```python
from build123d import *

# Parameters (mm, degrees)
CROQUIS1_W     = 15
CROQUIS1_H     = 65
EXTRUIR1_DEPTH = 6
CROQUIS2_W     = 15
CROQUIS2_H     = 6
EXTRUIR2_DEPTH = 50
CHAFL_N1_SIZE  = 2
CROQUIS3_R     = 4
EXTRUIR3_DEPTH = 50
CHAFL_N2_SIZE  = 3
REDONDEO1_R    = 6
CROQUIS4_R     = 4
EXTRUIR4_DEPTH = 30
REDONDEO2_R    = 0.5
EXTRUIR5_DEPTH = 15
CHAFL_N3_SIZE  = 9
EXTRUIR6_DEPTH = 15
CHAFL_N4_SIZE  = 3


with BuildPart() as part:
    # Croquis1 → Extruir1 (new body)
    with BuildSketch(Plane.XY):
        Rectangle(CROQUIS1_W, CROQUIS1_H)
    extrude(amount=EXTRUIR1_DEPTH)

    # Croquis2 → Extruir2 (add)
    with BuildSketch(Plane(origin=(0, 0, 0), x_dir=(-1, 0, 0), z_dir=(0, 0, -1))):
        with Locations((0, 29.5)):
            Rectangle(CROQUIS2_W, CROQUIS2_H)
    extrude(amount=EXTRUIR2_DEPTH)

    # Chaflán1
    chafl_n1_edges = [part.edges().sort_by_distance(p)[0] for p in [
        (0, 32.5, 6),
        (0, 26.5, 0),
    ]]
    chamfer(chafl_n1_edges, length=CHAFL_N1_SIZE)

    # Croquis3 → Extruir3 (add)
    with BuildSketch(Plane(origin=(0, 0, 0), x_dir=(-1, 0, 0), z_dir=(0, 0, -1))):
        with Locations(Location((0, -25.5, 0), (0, 0, 180))):
            Circle(CROQUIS3_R)
    extrude(amount=EXTRUIR3_DEPTH)

    # Chaflán2
    chafl_n2_edges = [part.edges().sort_by_distance(p)[0] for p in [
        (-4, -25.5, 0),
    ]]
    chamfer(chafl_n2_edges, length=CHAFL_N2_SIZE - 0.0001)  # a hair under: the kernel refuses the full size

    # Redondeo1
    redondeo1_edges = [part.edges().sort_by_distance(p)[0] for p in [
        (-7.5, -32.5, 3),
        (7.5, -32.5, 3),
    ]]
    fillet(redondeo1_edges, radius=REDONDEO1_R)

    # Croquis4 → Extruir4 (add)
    with BuildSketch(Plane(origin=(0, 32.5, 0), x_dir=(1, 0, 0), z_dir=(0, 1, 0))):
        with Locations(Location((0, 23, 0), (0, 0, 90))):
            Circle(CROQUIS4_R)
    extrude(amount=EXTRUIR4_DEPTH)

    # Redondeo2
    redondeo2_edges = [part.edges().sort_by_distance(p)[0] for p in [
        (0, 32.5, -19),
    ]]
    fillet(redondeo2_edges, radius=REDONDEO2_R)

    # Croquis6 → Extruir5 (add)
    with BuildSketch(Plane.XY.offset(6)):
        with BuildLine():
            Line((7.5, 0), (-7.5, 0))
            Line((-7.5, 0), (-7.5, -26.5))
            ThreePointArc((-7.5, -26.5), (-5.742640687, -30.742640687), (-1.5, -32.5))
            Line((-1.5, -32.5), (1.5, -32.5))
            ThreePointArc((1.5, -32.5), (5.742640687, -30.742640687), (7.5, -26.5))
            Line((7.5, -26.5), (7.5, 0))
        make_face()
    extrude(amount=-EXTRUIR5_DEPTH)

    # Chaflán3
    chafl_n3_edges = [part.edges().sort_by_distance(p)[0] for p in [
        (0, 0, 0),
    ]]
    chamfer(chafl_n3_edges, length=CHAFL_N3_SIZE - 0.0001)  # a hair under: the kernel refuses the full size

    # Croquis7 → Extruir6 (cut)
    with BuildSketch(Plane(origin=(7.5, 0, 0), x_dir=(0, 0, -1), z_dir=(1, 0, 0))):
        Polygon((-6, 6.514718626), (3, -2.485281374), (3, -32.5), (-11.901527466, -39.580751492), align=None)
    extrude(amount=-EXTRUIR6_DEPTH, mode=Mode.SUBTRACT)

    # Chaflán4
    chafl_n4_edges = [part.edges().sort_by_distance(p)[0] for p in [
        (-4, -25.5, -9),
    ]]
    chamfer(chafl_n4_edges, length=CHAFL_N4_SIZE - 0.0001)  # a hair under: the kernel refuses the full size


solid = part.part
```
Check sheet for the modelled part. Datum: model origin and axes. Units: mm. A direction names the side the tool comes from. Coordinates: 2 decimals unless noted, no trailing zeros. Loops run counter-clockwise (first coordinate to the right, second up) from the corner with the lowest first, then second, coordinate; pieces in that order, holes last.
1) Release check for a two-part mould opening along Y. For faces 1 (the face through (0, 4, -5)), 2 (the face through (0, 62.5, -23)), 3 (the face through (-0.54, -21.39, -11.854)), 4 (the face through (-7.5, 27, -11)) record: released by +Y, released by -Y, zero draft, split by the parting line, or undercut.
2) Gauge pin test, flat ends, axial feed: pin 1 (4.5 mm diameter, centred on x = -2.5, y = -12, fed in from -Z); pin 2 (7.5 mm diameter, centred on x = 2.5, y = -20, fed in from +Z); pin 3 (4 mm diameter, centred on x = 1, z = -39, fed in from +Y); pin 4 (2 mm diameter, centred on y = 34, z = -17.5, fed in from +X). Record the tip position at first contact, or that the pin passes through.
3) Sectioned sample at D-D (z = -37). Record the boundary of the cut face in (x, y).
4) Material ranges on probe 1 along Z at (x, y) = (-4, -13); probe 2 along Y at (x, z) = (3.5, -34); probe 3 along Y at (x, z) = (-0.5, -10.5), recorded low to high.
5) Sectioned sample at C-C (y = -25.5). Record the boundary of the cut face in (x, z).
6) Sectioned sample at A-A (z = -23). Record the boundary of the cut face in (x, y), and give its area (3 significant figures).
7) Access from +Z, -Z, +X, -X, +Y, -Y to the whole of each face (thin tool, end or side, straight path). Record for faces 5 (the face through (0, -17, -3)), 6 (the face through (-0.521, -29.466, -30.734)), 7 (the face through (2.4, 47.5, -19.8)), 8 (the face through (0, 30, -50)), 9 (the face through (0.1, 25.5, -1)).
Check sheet entries:
1. face 1: undercut
1. face 2: released by +Y
1. face 3: undercut
1. face 4: zero draft
2. pin 1: stops at z = -9
2. pin 2: stops at z = -3
2. pin 3: stops at y = 32.5
2. pin 4: passes through
3. outline: (-7.5, 26.5) - (7.5, 26.5) - (7.5, 32.5) - (-7.5, 32.5) - close; circle Ø8 at (0, -25.5)
4. probe 1: z = -9 to -3
4. probe 2: y = -27.44 to -23.56, 26.5 to 32.5
4. probe 3: y = -30.98 to -20.02, 26.5 to 32.5
5. outline: (-7.5, -9) - (-7, -9) - (-4, -12) - (-4, -50) - (4, -50) - (4, -12) - (7, -9) - (7.5, -9) - (7.5, -3) - (-7.5, -3) - close
6. outline: (-7.5, 26.5) - (7.5, 26.5) - (7.5, 32.5) - (4.5, 32.5) arc R0.5 cw to (4, 33) - (4, 62.5) - (-4, 62.5) - (-4, 33) arc R0.5 cw to (-4.5, 32.5) - (-7.5, 32.5) - close; circle Ø8 at (0, -25.5)
6. area: 380 mm2
7. face 5: +Z, +X, -X, -Y
7. face 6: -Z
7. face 7: +Y
7. face 8: -Z, +X, -X, +Y, -Y
7. face 9: -Z, +X, -X
